```python
from build123d import *

# Parameters (mm, degrees)
F0_R     = 1.905
F0_R_2   = 1.27
F1_DEPTH = 12.7
F2_W     = 2.032
F2_H     = 13.7110514179
F3_DEPTH = 12.7
F5_DEPTH = 1.27


with BuildPart() as f1:
    # F0 (on Top) → F1 (new body)
    with BuildSketch(Plane.XY):
        Circle(F0_R)
        Circle(F0_R_2, mode=Mode.SUBTRACT)
    extrude(amount=F1_DEPTH)

    # F2 (on Front) → F3 (cut, symmetric)
    with BuildSketch(Plane.XZ):
        with Locations((0, 13.2055257089)):
            Rectangle(F2_W, F2_H)
    extrude(amount=F3_DEPTH, both=True, mode=Mode.SUBTRACT)

    # F4 (on face) → F5 (join)
    with BuildSketch(Plane.XY.offset(6.35)):
        with BuildLine():
            Line((-1.016, 1.6114493476), (-1.016, -1.6114493476))
            ThreePointArc((-1.016, -1.6114493476), (0, -1.905), (1.016, -1.6114493476))
            Line((1.016, -1.6114493476), (1.016, 1.6114493476))
            ThreePointArc((1.016, 1.6114493476), (0, 1.905), (-1.016, 1.6114493476))
        make_face()
    extrude(amount=F5_DEPTH)


solid = f1.part
```
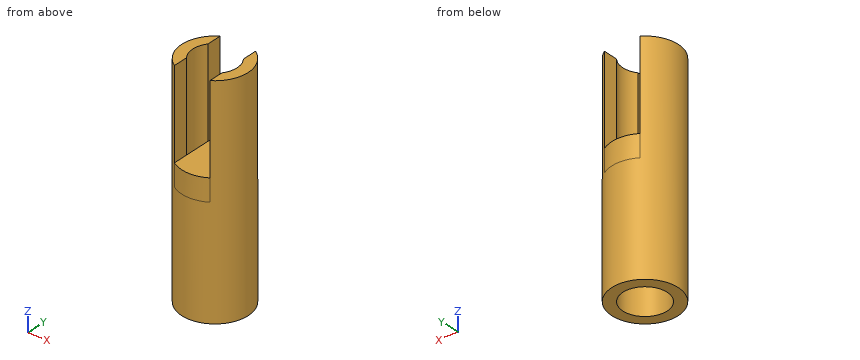
Model file for the job. Use its own axes, mm. Coordinates: 2 decimals unless noted, no trailing zeros. Write each loop counter-clockwise with the first axis right and the second up, starting at its lowest first coordinate (ties: lowest second). Pieces come first, ordered by that corner, then holes. Notation, with made-up numbers: (65, 37) - (120, 37) arc R24 cw to (120, 73) - close; hole circle Ø9 at (60.5, -13.75). An arc over 180 degrees is marked (long way). One line per item, written item: value. Start each with the question number.
1. Flat gauge pins, fed straight in: pin 1 (1 mm diameter, centred on x = 0, y = -0.5, fed in from -Z); pin 2 (0.9 mm diameter, centred on y = -1, z = 9.5, fed in from -X); pin 3 (0.9 mm diameter, centred on y = 1.5, z = 10, fed in from +X). Where does each tip first touch, or does it go through?
2. Probe line 1 (X direction, y = 0, z = 7) (3 decimals); line 2 (X direction, y = 0, z = 10) (3 decimals). List the from-to ranges inside material, lowest first. Write a range as from..to.
3. Slice it at C-C (x = -1.15). Write the cut outline in (y, z).
4. Slice it at D-D (x = 0). Write the cut outline in (y, z) (3 decimals).
5. Slice it at A-A (z = 11.25). Write the cut outline in (x, y) (3 decimals), plus the area to 3 significant figures.
6. Slice it at B-B (y = 0). Write the cut outline in (x, z) (3 decimals).
Answers below:
1. pin 1: stops at z = 6.35
1. pin 2: stops at x = -1.82
1. pin 3: stops at x = 1.59
2. line 1: x = -1.905..-1.27, -1.016..1.016, 1.27..1.905
2. line 2: x = -1.905..-1.27, 1.27..1.905
3. outline: (-1.52, 0) - (-0.54, 0) - (-0.54, 12.7) - (-1.52, 12.7) - close; (0.54, 0) - (1.52, 0) - (1.52, 12.7) - (0.54, 12.7) - close
4. outline: (-1.905, 0) - (-1.27, 0) - (-1.27, 6.35) - (1.27, 6.35) - (1.27, 0) - (1.905, 0) - (1.905, 7.62) - (-1.905, 7.62) - close
5. outline: (-1.016, -1.611) - (-1.016, -0.762) arc R1.27 cw to (-1.016, 0.762) - (-1.016, 1.611) arc R1.905 ccw to start; (1.016, -1.611) arc R1.905 ccw to (1.016, 1.611) - (1.016, 0.762) arc R1.27 cw to (1.016, -0.762) - close
5. area: 3.52 mm^2
6. outline: (-1.905, 0) - (-1.27, 0) - (-1.27, 12.7) - (-1.905, 12.7) - close; (-1.016, 6.35) - (1.016, 6.35) - (1.016, 7.62) - (-1.016, 7.62) - close; (1.27, 0) - (1.905, 0) - (1.905, 12.7) - (1.27, 12.7) - close
